The model under review builds one solid part; all positions refer to its coordinate system, in mm. A direction names the side the tool comes from. Give positions to 0.01 mm unless a question says otherwise; leave off trailing zeros. Order: outer loops, then holes, each group sorted by start corner. A loop starts at its lowest first (then second) coordinate and runs counter-clockwise, first axis right, second up. Notation, with made-up numbers: (-39, 51) - (-18, 51) arc R29 cw to (-18, 71) - close; hole circle Ø8 at (89.5, 48.5). An arc over 180 degrees is marked (long way). Put each result on its own line as item: value.
```python
from build123d import *

# Parameters (mm, degrees)
SKETCH1_W           = 20
SKETCH1_H           = 4
BOSS_EXTRUDE1_DEPTH = 8
SKETCH2_W           = 7
SKETCH2_H           = 2
CUT_EXTRUDE1_DEPTH  = 8
SKETCH3_W           = 8
SKETCH3_H           = 4
BOSS_EXTRUDE2_DEPTH = 10
SKETCH4_R           = 1.5
CUT_EXTRUDE2_DEPTH  = 10
CUT_EXTRUDE3_DEPTH  = 2


with BuildPart() as part:
    # Sketch1 → Boss-Extrude1 (new body)
    with BuildSketch(Plane.XY):
        with Locations((10, 2)):
            Rectangle(SKETCH1_W, SKETCH1_H)
    extrude(amount=BOSS_EXTRUDE1_DEPTH)

    # Sketch2 → Cut-Extrude1 (cut)
    with BuildSketch(Plane.XY.offset(8)):
        with Locations((5.5, 3)):
            Rectangle(SKETCH2_W, SKETCH2_H)
    extrude(amount=-CUT_EXTRUDE1_DEPTH, mode=Mode.SUBTRACT)

    # Sketch3 → Boss-Extrude2 (add)
    with BuildSketch(Plane(origin=(20, 0, 0), x_dir=(0, 0, -1), z_dir=(1, 0, 0))):
        with Locations((-4, 2)):
            Rectangle(SKETCH3_W, SKETCH3_H)
    extrude(amount=BOSS_EXTRUDE2_DEPTH)

    # Sketch4 → Cut-Extrude2 (cut)
    with BuildSketch(Plane.XZ):
        with Locations(Location((25, 4, 0), (0, 0, 270))):
            Circle(SKETCH4_R)
        with Locations(Location((15, 4, 0), (0, 0, 270))):
            Circle(SKETCH4_R)
    extrude(amount=-CUT_EXTRUDE2_DEPTH, mode=Mode.SUBTRACT)

    # Sketch5 → Cut-Extrude3 (cut)
    with BuildSketch(Plane.XZ):
        Polygon((22, 4), (23.5, 1.401923789), (26.5, 1.401923789), (28, 4), (26.5, 6.598076211), (23.5, 6.598076211), align=None)
        Polygon((12, 4), (13.5, 1.401923789), (16.5, 1.401923789), (18, 4), (16.5, 6.598076211), (13.5, 6.598076211), align=None)
    extrude(amount=-CUT_EXTRUDE3_DEPTH, mode=Mode.SUBTRACT)


solid = part.part
```
(1) Take a section at C-C, the plane y = 0.8. Write out the cut boundary in (x, z).
The answers:
outline: (0, 0) - (30, 0) - (30, 8) - (0, 8) - close; hole (12, 4) - (13.5, 1.4) - (16.5, 1.4) - (18, 4) - (16.5, 6.6) - (13.5, 6.6) - close; hole (22, 4) - (23.5, 1.4) - (26.5, 1.4) - (28, 4) - (26.5, 6.6) - (23.5, 6.6) - close
(2) Take a section at B-B, the plane x = 15. Write out the cut boundary in (y, z).
The answers:
outline: (0, 0) - (4, 0) - (4, 2.5) - (2, 2.5) - (2, 1.4) - (0, 1.4) - close; (0, 6.6) - (2, 6.6) - (2, 5.5) - (4, 5.5) - (4, 8) - (0, 8) - close
(3) Take a section at D-D, the plane z = 4.5. Write out the cut boundary in (x, y).
The answers:
outline: (0, 0) - (12.29, 0) - (12.29, 2) - (13.59, 2) - (13.59, 4) - (9, 4) - (9, 2) - (2, 2) - (2, 4) - (0, 4) - close; (16.41, 2) - (17.71, 2) - (17.71, 0) - (22.29, 0) - (22.29, 2) - (23.59, 2) - (23.59, 4) - (16.41, 4) - close; (26.41, 2) - (27.71, 2) - (27.71, 0) - (30, 0) - (30, 4) - (26.41, 4) - close
(4) Take a section at A-A, the plane y = 3.7. Write out the cut boundary in (x, z).
The answers:
outline: (0, 0) - (2, 0) - (2, 8) - (0, 8) - close; (9, 0) - (30, 0) - (30, 8) - (9, 8) - close; hole circle Ø3 at (15, 4); hole circle Ø3 at (25, 4)
(5) Wall thickness on L1, parallel to X at y = 3.4, z = 4; L2, parallel to X at y = 3, z = 7; L3, parallel to X at y = 1.35, z = 3: over which ranges is each line inside the solid? List them lowest first.
The answers:
L1: 0 to 2, 9 to 13.5, 16.5 to 23.5, 26.5 to 30
L2: 0 to 2, 9 to 30
L3: 0 to 12.58, 17.42 to 22.58, 27.42 to 30
(6) Clearance check with flat-ended pins moving along their axes: pin 1 Ø4 at (x, z) = (15, 4) entering from -Y; pin 2 Ø0.6 at (x, y) = (25.5, 0.5) entering from -Z; pin 3 Ø2.5 at (x, z) = (25, 4) entering from +Y. State where each tip first meets the part, or that it passes through.
The answers:
pin 1: y = 2
pin 2: z = 0
pin 3: through
(7) For faces 3 (the flat face through (25, 1, 6.598)), 4 (the flat face through (15, 2, 0)), 5 (the flat face through (5, 2, 4)), list the 3-axis set-ups (+Z, -Z, +X, -X, +Y, -Y) from which the entire face can be reached by the end or side of a thin tool; tool diameter is ignored.
The answers:
face 3: -Y
face 4: -Z, +X, -X, +Y, -Y
face 5: +Z, -Z, +Y
(8) The part is to be moulded in two halves that separate along X. For faces 1 (the cylindrical face through (26.487, 2.986, 4.195)), 2 (the flat face through (1, 4, 4)), say which applies: pulls with the +X half, pulls with the -X half, needs draft (parallel to the pull), parting line crosses it, or undercut.
The answers:
face 1: undercut
face 2: needs draft
